Design review of the part built by this model. Coordinates are the model's own, in mm. Coordinates: 2 decimals unless noted, no trailing zeros. Write each loop counter-clockwise with the first axis right and the second up, starting at its lowest first coordinate (ties: lowest second). Pieces come first, ordered by that corner, then holes. Notation, with made-up numbers: (74.5, -34.75) - (107.5, -34.75) arc R22 ccw to (107.5, 3.25) - close; hole circle Ø7 at (73, -33.5). An arc over 180 degrees is marked (long way). Answer as CSV lines item,"result". Start each with the question number.
Q1. We need section C-C (y = 85.5). Write out the cut boundary in (x, z), plus the area to 3 significant figures.
Q2. Clearance check with flat-ended pins moving along their axes: pin 1 (4 mm diameter, centred on y = 105, z = -40, fed in from +X); pin 2 (12 mm diameter, centred on x = -12, y = 235, fed in from -Z); pin 3 (12 mm diameter, centred on y = 261.5, z = 29, fed in from +X). State where each tip first meets the part, or that it passes through.
Q3. Mouldability with a two-part tool opening along Z and no side actions: class faces 1 (the face through (47.24, 300.53, -14.88)), 2 (the face through (-11.012, 300.533, 49.592)), 3 (the face through (11, 609.6, 49)) as pulls with the +Z half, pulls with the -Z half, needs draft (parallel to the pull), parting line crosses it, or undercut.
Q4. We need section B-B (x = 31). Write out the cut boundary in (y, z).
Q5. For line 1 along Z through (x, y) = (0, 231.5); line 2 along X through (y, z) = (390, -13), list the stretches that pass through material, from the lowest coordinate up. Write a range as [from, to].
Q6. We need section A-A (z = -15). Write out the cut boundary in (x, y).
from build123d import *

# Parameters (mm, degrees)
SKETCH1_R           = 50.8
SKETCH1_R_2         = 49.53
BOSS_EXTRUDE1_DEPTH = 609.6
SKETCH2_R           = 1.984375
CUT_EXTRUDE1_DEPTH  = 12.7
CIRPATTERN1_COUNT   = 4


with BuildPart() as part:
    # Sketch1 → Boss-Extrude1 (new body)
    with BuildSketch(Plane(origin=(0, 0, 0), x_dir=(1, 0, 0), z_dir=(0, 1, 0))):
        Circle(SKETCH1_R)
        Circle(SKETCH1_R_2, mode=Mode.SUBTRACT)
    extrude(amount=BOSS_EXTRUDE1_DEPTH)

    # Sketch2 → Cut-Extrude1 (cut)
    with BuildSketch(Plane(origin=(122.899951256, 815.595371644, -42.551362721), x_dir=(-0.997691035, 0, -0.067916112), z_dir=(0.067916112, 0, -0.997691035))):
        with Locations((119.72625647, -256.795371644)):
            Circle(SKETCH2_R)
    cut_extrude1 = extrude(amount=-CUT_EXTRUDE1_DEPTH, mode=Mode.SUBTRACT)

    # CirPattern1: Cut-Extrude1 ×4 about axis
    cirpattern1_axis = Axis((0, 0, 0), (0, -1, 0))
    for i in range(1, CIRPATTERN1_COUNT):
        add(cut_extrude1.rotate(cirpattern1_axis, i * 360 / CIRPATTERN1_COUNT), mode=Mode.SUBTRACT)


solid = part.part
Results list:
1,outline,"circle Ø101.6 at (0, 0); hole circle Ø99.06 at (0, 0)"
1,area,"400 mm2"
2,pin 1,"stops at x = 33.71"
2,pin 2,"stops at z = -50.44"
2,pin 3,"stops at x = 45.3"
3,face 1,"undercut"
3,face 2,"parting line crosses it"
3,face 3,"needs draft"
4,outline,"(0, -40.24) - (609.6, -40.24) - (609.6, -38.63) - (0, -38.63) - close; (0, 38.63) - (609.6, 38.63) - (609.6, 40.24) - (0, 40.24) - close"
5,line 1,"z = [-50.8, -49.53], [49.53, 50.8]"
5,line 2,"x = [-49.11, -47.79], [47.79, 49.11]"
6,outline,"(-48.53, 0) - (-47.2, 0) - (-47.2, 609.6) - (-48.53, 609.6) - close; (47.2, 0) - (48.53, 0) - (48.53, 609.6) - (47.2, 609.6) - close"
